Part print with two shaded views. Sizes in mm from the minimum x, y, z corner. Round coordinates to 2 decimals unless told otherwise and drop trailing zeros. Loops run counter-clockwise (first coordinate to the right, second up) from the corner with the lowest first, then second, coordinate; pieces in that order, holes last. Notation, with made-up numbers: (-23.75, -29.75) -> (33.25, -29.75) arc R17 ccw to (33.25, -8.75) -> close; hole circle Ø3 at (38.25, 41). An arc over 180 degrees is marked (long way). Answer as a JSON object with one key per item and string values. Group by question number.
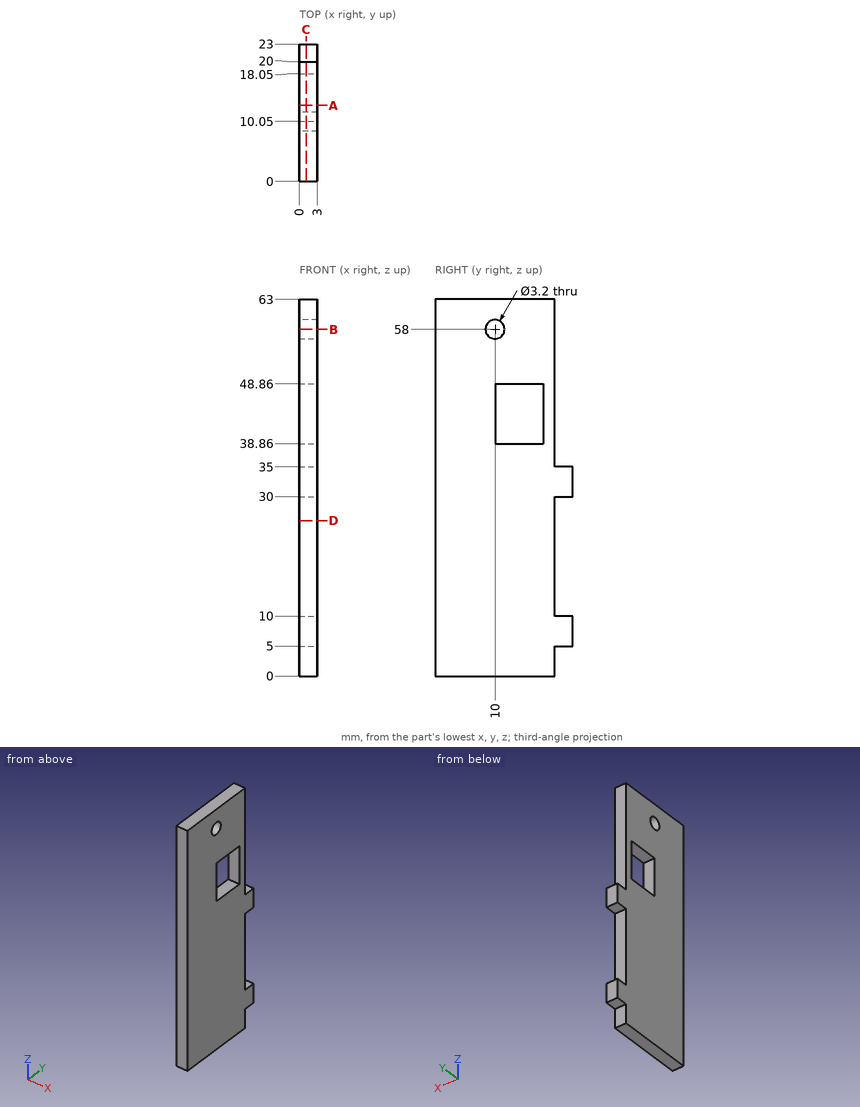
Item 1: Drill centre lines: line 1 (Y direction, x = 2.4, z = 40); line 2 (Y direction, x = 1.3, z = 58); line 3 (Z direction, x = 1.15, y = 14). Where is each one in solid material? Low to high.
Item 2: Band-saw the part on B-B, the plane z = 58. List the corners of the cut face in (x, y).
Item 3: Drop a flat-ended pin along its axis: pin 1 Ø1.5 at (x, z) = (1, 21.5) entering from +Y. Give the stop position or say it passes through.
Item 4: Band-saw the part on A-A, the plane y = 12.75. List the corners of the cut face in (x, z), plus the area to 3 significant figures.
Item 5: Band-saw the part on C-C, the plane x = 1.15. List the corners of the cut face in (y, z).
Item 6: Band-saw the part on D-D, the plane z = 26. List the corners of the cut face in (x, y).
Entries:
{
 "1": {"line 1": "0 to 10.05, 18.05 to 20", "line 2": "0 to 8.4, 11.6 to 20", "line 3": "0 to 38.86, 48.86 to 63"},
 "2": {"outline": "(0, 0) -> (3, 0) -> (3, 8.4) -> (0, 8.4) -> close; (0, 11.6) -> (3, 11.6) -> (3, 20) -> (0, 20) -> close"},
 "3": {"pin 1": "y = 20"},
 "4": {"outline": "(0, 0) -> (3, 0) -> (3, 38.86) -> (0, 38.86) -> close; (0, 48.86) -> (3, 48.86) -> (3, 63) -> (0, 63) -> close", "area": "159 mm²"},
 "5": {"outline": "(0, 0) -> (20, 0) -> (20, 5) -> (23, 5) -> (23, 10) -> (20, 10) -> (20, 30) -> (23, 30) -> (23, 35) -> (20, 35) -> (20, 63) -> (0, 63) -> close; hole circle Ø3.2 at (10, 58); hole (10.05, 38.86) -> (18.05, 38.86) -> (18.05, 48.86) -> (10.05, 48.86) -> close"},
 "6": {"outline": "(0, 0) -> (3, 0) -> (3, 20) -> (0, 20) -> close"}
}
